from build123d import *


with BuildPart() as part:
    # Croquis1 → Revolución1 (revolve)
    with BuildSketch(Plane(origin=(0, 0, 0), x_dir=(-1, 0, 0), z_dir=(0, 1, 0)), mode=Mode.PRIVATE) as revoluci_n1_sk:
        Polygon((-17.4, 3), (17.4, 3), (17.4, 2.55), (18.2, 2.55), (18.2, 3), (22.4, 3), (22.4, 0), (-22.4, 0), (-22.4, 3), (-18.2, 3), (-18.2, 2.55), (-17.4, 2.55), align=None)
    revolve(revoluci_n1_sk.sketch.rotate(Axis((22.4, 0, 0), (-1, 0, 0)), 180), axis=Axis((22.4, 0, 0), (-1, 0, 0)))


solid = part.part
Verification items for the finished model (mm, model axes). A direction names the side the tool comes from. Coordinates: 2 decimals unless noted, no trailing zeros. Order: outer loops, then holes, each group sorted by start corner. A loop starts at its lowest first (then second) coordinate and runs counter-clockwise, first axis right, second up. Notation, with made-up numbers: (8.25, 27) -> (38.25, 27) arc R18 cw to (38.25, 31) -> close; hole circle Ø4 at (49, 26.5). An arc over 180 degrees is marked (long way). Use CSV: the item, a comma, the result in double quotes. Start each with the question number.
Q1. Section check C-C, the plane x = 1.5. Record the cut outline in (y, z).
Q2. Thickness scan on line 1 along X through (y, z) = (-2.8, -0.3); line 2 along Y through (x, z) = (-19, 0.2); line 3 along Z through (x, y) = (13.5, -1.75). Record the ranges inside material, lowest first.
Q3. Section check A-A, the plane z = 1.8. Record the cut outline in (x, y).
Q4. Depth check by flat-ended pin: P1, Ø2, axis at x = -12.5, z = 2, coming from the +Y side. Enter the tip coordinate at first touch or a pass-through.
Q5. Tool access check on faces 1 (the flat face through (18.2, -2, 2)), 2 (the cylindrical face through (20.27, -0.9, -2.86)). Record the directions out of +Z, -Z, +X, -X, +Y, -Y that give a thin tool (end or side, any length) a straight path to the whole face; none if there is none.
Returned:
1,outline,"circle Ø6 at (0, 0)"
2,line 1,"x = -22.4 to -18.2, -17.4 to 17.4, 18.2 to 22.4"
2,line 2,"y = -2.99 to 2.99"
2,line 3,"z = -2.44 to 2.44"
3,outline,"(-22.4, -2.4) -> (-18.2, -2.4) -> (-18.2, -1.81) -> (-17.4, -1.81) -> (-17.4, -2.4) -> (17.4, -2.4) -> (17.4, -1.81) -> (18.2, -1.81) -> (18.2, -2.4) -> (22.4, -2.4) -> (22.4, 2.4) -> (18.2, 2.4) -> (18.2, 1.81) -> (17.4, 1.81) -> (17.4, 2.4) -> (-17.4, 2.4) -> (-17.4, 1.81) -> (-18.2, 1.81) -> (-18.2, 2.4) -> (-22.4, 2.4) -> close"
4,P1,"stops at y = 2.83"
5,face 1,"none"
5,face 2,"+X, -X"
